Input: part model. Units: mm. Frame: model coordinates. Face numbers are marked on the shaded views. A direction names the side the tool comes from. Give positions to 0.01 mm unless a question says otherwise; leave off trailing zeros. Loops run counter-clockwise (first coordinate to the right, second up) from the corner with the lowest first, then second, coordinate; pieces in that order, holes last. Notation, with made-up numbers: M 55.25,42.25 L 75.25,42.25 A26 cw 75.25,65.25 Z; hole C -6.5,79.25 d5. An arc over 180 degrees is marked long. Use a Markdown table: item, result. Add a question column.
from build123d import *

# Parameters (mm, degrees)
BOSS_EXTRUDE1_DEPTH  = 32.5
SKETCH4_R            = 1.05
BOSS_EXTRUDE2_DEPTH  = 2
SKETCH7_R            = 2.495
WIRE_SPACING2_DEPTH  = 3
SKETCH8_W            = 35
SKETCH8_H            = 37.7
SKETCH8_R            = 2.495
BOSS_EXTRUDE6_DEPTH  = 2
SKETCH5_R            = 1.05
BOSS_EXTRUDE3_DEPTH  = 2
SKETCH9_R            = 2.495
WIRE_SPACING1_DEPTH  = 3
SKETCH10_W           = 35
SKETCH10_H           = 37.7
SKETCH10_R           = 2.495
BOSS_EXTRUDE8_DEPTH  = 2
SKETCH11_R           = 12.5
CUT_EXTRUDE1_DEPTH   = 47.5
CUT_EXTRUDE2_DEPTH   = 47.5
SKETCH13_W           = 45
SKETCH13_H           = 46.5
BOSS_EXTRUDE9_DEPTH  = 17.5
SKETCH15_W           = 12.5
SKETCH15_H           = 46.5
BOSS_EXTRUDE10_DEPTH = 50
SKETCH18_R           = 4
SKETCH18_R_2         = 1.7
BOSS_EXTRUDE11_DEPTH = 46.5
BOSS_EXTRUDE13_DEPTH = 46.5
SKETCH21_W           = 89.912502986
SKETCH21_H           = 37.65
CUT_EXTRUDE3_DEPTH   = 46
CUT_EXTRUDE5_DEPTH   = 47.5
CUT_EXTRUDE4_START   = -50.5000001
CUT_EXTRUDE4_DEPTH   = 101.5000002
CUT_EXTRUDE6_DEPTH   = 53.0000001
BOSS_EXTRUDE14_DEPTH = 46.5
FILLET2_R            = 10
SKETCH29_W           = 2.5
SKETCH29_H           = 42.5
CUT_EXTRUDE8_DEPTH   = 9.427041
FILLET3_R            = 1
SKETCH30_W           = 7.311581117
SKETCH30_H           = 8
CUT_EXTRUDE9_DEPTH   = 22.5


with BuildPart() as part:
    # Sketch2 → Boss-Extrude1 (new body)
    with BuildSketch(Plane(origin=(0, 0, 0), x_dir=(1, 0, 0), z_dir=(0, 1, 0))):
        Polygon((17.5, 0), (17.5, 37.7), (15, 37.7), (15, 2.5), (-15, 2.5), (-15, 37.7), (-17.5, 37.7), (-17.5, 0), align=None)
    extrude(amount=BOSS_EXTRUDE1_DEPTH)

    # Sketch4 → Boss-Extrude2 (add)
    with BuildSketch(Plane.XZ):
        Polygon((-17.5, 0), (-17.5, -7.443777264), (-17.5, -37.7), (-15, -37.7), (-15, -7.5), (15, -7.5), (15, -37.7), (17.5, -37.7), (17.5, -7.443777264), (17.5, 0), align=None)
        with Locations((-10.1889, -4.95)):
            Circle(SKETCH4_R, mode=Mode.SUBTRACT)
        with Locations((10.1889, -4.95)):
            Circle(SKETCH4_R, mode=Mode.SUBTRACT)
    extrude(amount=BOSS_EXTRUDE2_DEPTH)

    # Sketch7 → Wire spacing2 (add)
    with BuildSketch(Plane.XZ.offset(2)):
        Polygon((-17.5, 0), (-17.5, -37.7), (-15, -37.7), (-15, -7.5), (15, -7.5), (15, -37.7), (17.5, -37.7), (17.5, 0), align=None)
        with Locations((-10.1889, -4.95)):
            Circle(SKETCH7_R, mode=Mode.SUBTRACT)
        with Locations((10.1889, -4.95)):
            Circle(SKETCH7_R, mode=Mode.SUBTRACT)
    extrude(amount=WIRE_SPACING2_DEPTH)

    # Sketch8 → Boss-Extrude6 (add)
    with BuildSketch(Plane.XZ.offset(5)):
        with Locations((0, -18.85)):
            Rectangle(SKETCH8_W, SKETCH8_H)
        with Locations((-10.1889, -4.95)):
            Circle(SKETCH8_R, mode=Mode.SUBTRACT)
        with Locations((10.1889, -4.95)):
            Circle(SKETCH8_R, mode=Mode.SUBTRACT)
    extrude(amount=BOSS_EXTRUDE6_DEPTH)

    # Sketch5 → Boss-Extrude3 (add)
    with BuildSketch(Plane(origin=(0, 32.5, 0), x_dir=(1, 0, 0), z_dir=(0, 1, 0))):
        Polygon((-7.439, 10), (-7.439, 2.5), (7.439, 2.5), (7.439, 10), (10.1889, 12), (15, 12), (15, 37.7), (17.5, 37.7), (17.5, 0), (-17.5, 0), (-17.5, 37.7), (-15, 37.7), (-15, 12), (-10.1889, 12), align=None)
        with Locations((-10.1889, 8.7)):
            Circle(SKETCH5_R, mode=Mode.SUBTRACT)
        with Locations((10.1889, 8.7)):
            Circle(SKETCH5_R, mode=Mode.SUBTRACT)
    extrude(amount=BOSS_EXTRUDE3_DEPTH)

    # Sketch9 → Wire spacing1 (add)
    with BuildSketch(Plane(origin=(0, 34.5, 0), x_dir=(1, 0, 0), z_dir=(0, 1, 0))):
        Polygon((-17.5, 0), (-17.5, 37.7), (-15, 37.7), (-15, 12), (-10.1889, 12), (-7.439, 10), (-7.439, 2.5), (7.439, 2.5), (7.439, 10), (10.1889, 12), (15, 12), (15, 37.7), (17.5, 37.7), (17.5, 0), align=None)
        with Locations((-10.1889, 8.7)):
            Circle(SKETCH9_R, mode=Mode.SUBTRACT)
        with Locations((10.1889, 8.7)):
            Circle(SKETCH9_R, mode=Mode.SUBTRACT)
    extrude(amount=WIRE_SPACING1_DEPTH)

    # Sketch10 → Boss-Extrude8 (add)
    with BuildSketch(Plane(origin=(0, 37.5, 0), x_dir=(1, 0, 0), z_dir=(0, 1, 0))):
        with Locations((0, 18.85)):
            Rectangle(SKETCH10_W, SKETCH10_H)
        with Locations((-10.1889, 8.7)):
            Circle(SKETCH10_R, mode=Mode.SUBTRACT)
        with Locations((10.1889, 8.7)):
            Circle(SKETCH10_R, mode=Mode.SUBTRACT)
    extrude(amount=BOSS_EXTRUDE8_DEPTH)

    # Sketch11 → Cut-Extrude1 (cut, through all)
    with BuildSketch(Plane(origin=(0, 39.5, 0), x_dir=(1, 0, 0), z_dir=(0, 1, 0))):
        with Locations((0, 37.7)):
            Circle(SKETCH11_R)
    extrude(amount=-CUT_EXTRUDE1_DEPTH, mode=Mode.SUBTRACT)

    # Sketch12 → Cut-Extrude2 (cut, through all)
    with BuildSketch(Plane.XZ.offset(7)):
        Polygon((0, -25.2), (17.5, -15), (17.5, -47.484525272), align=None)
    extrude(amount=-CUT_EXTRUDE2_DEPTH, mode=Mode.SUBTRACT)

    # Sketch13 → Boss-Extrude9 (add)
    with BuildSketch(Plane.XY):
        with Locations((-5, 16.25)):
            Rectangle(SKETCH13_W, SKETCH13_H)
    extrude(amount=BOSS_EXTRUDE9_DEPTH)

    # Sketch15 → Boss-Extrude10 (add)
    with BuildSketch(Plane(origin=(0, 0, 0), x_dir=(-1, 0, 0), z_dir=(0, 0, -1))):
        with Locations((21.25, 16.25)):
            Rectangle(SKETCH15_W, SKETCH15_H)
    extrude(amount=BOSS_EXTRUDE10_DEPTH)

    # Sketch18 → Boss-Extrude11 (add)
    with BuildSketch(Plane.XZ.offset(7)):
        with BuildLine():
            Line((12.5, 22.5), (12.5, 17.5))
            Line((12.5, 17.5), (-12.5, 17.5))
            Line((-12.5, 17.5), (-12.5, 22.5))
            Line((-12.5, 22.5), (-9.367496998, 30))
            ThreePointArc((-9.367496998, 30), (0, 49.5), (9.367496998, 30))
            Line((9.367496998, 30), (12.5, 22.5))
        make_face()
        with Locations((0, 37.5)):
            Circle(SKETCH18_R, mode=Mode.SUBTRACT)
        with Locations((0, 30.5)):
            Circle(SKETCH18_R_2, mode=Mode.SUBTRACT)
        with Locations((-7, 37.5)):
            Circle(SKETCH18_R_2, mode=Mode.SUBTRACT)
        with Locations((0, 44.5)):
            Circle(SKETCH18_R_2, mode=Mode.SUBTRACT)
        with Locations((7, 37.5)):
            Circle(SKETCH18_R_2, mode=Mode.SUBTRACT)
    extrude(amount=-BOSS_EXTRUDE11_DEPTH)

    # Sketch22 → Boss-Extrude13 (add)
    with BuildSketch(Plane.XZ.offset(7)):
        Polygon((-27.5, 17.5), (-5.066300312, 48.378078928), (-5.066300312, 17.5), align=None)
        Polygon((17.5, 17.5), (6.194336088, 47.777655396), (7.922300343, 17.5), align=None)
    extrude(amount=-BOSS_EXTRUDE13_DEPTH)

    # Sketch21 → Cut-Extrude3 (cut, through all)
    with BuildSketch(Plane.ZY.offset(27.5)):
        with Locations((62.456251493, 16.25)):
            Rectangle(SKETCH21_W, SKETCH21_H)
    extrude(amount=-CUT_EXTRUDE3_DEPTH, mode=Mode.SUBTRACT)

    # Sketch26 → Cut-Extrude5 (cut, through all)
    with BuildSketch(Plane(origin=(0, 39.5, 0), x_dir=(1, 0, 0), z_dir=(0, 1, 0))):
        with BuildLine():
            Line((-27.5, 29.387171818), (-27.5, 50))
            Line((-27.5, 50), (-15, 50))
            add(Edge.make_bspline(
                [(-15, 50), (-23.594741162, 41.153529081), (-27.5, 29.387171818)],
                knots=[0, 0, 0, 1, 1, 1], degree=2))
        make_face()
    extrude(amount=-CUT_EXTRUDE5_DEPTH, mode=Mode.SUBTRACT)

    # Sketch24 → Cut-Extrude4 (cut)
    with BuildSketch(Plane(origin=(0, 0, 0), x_dir=(-1, 0, 0), z_dir=(0, 0, -1)).offset(CUT_EXTRUDE4_START)):
        with BuildLine():
            Line((15, -7), (27.5, -7))
            Line((27.5, -7), (27.5, 16.25))
            add(Edge.make_bspline(
                [(27.5, 16.25), (23.398461901, 3.482399142), (15, -7)],
                knots=[0, 0, 0, 1, 1, 1], degree=2))
        make_face()
    cut_extrude4 = extrude(amount=CUT_EXTRUDE4_DEPTH, mode=Mode.SUBTRACT)

    # Mirror1: Cut-Extrude4 across plane
    add(cut_extrude4.mirror(Plane(origin=(0, 16.25, 0), x_dir=(0, 0, 1), z_dir=(0, -1, 0))), mode=Mode.SUBTRACT)

    # Sketch27 → Cut-Extrude6 (cut, through all)
    with BuildSketch(Plane(origin=(0, 0, -2.5), x_dir=(-1, 0, 0), z_dir=(0, 0, -1))):
        Polygon((-12.5, 26.25), (8.945069205, 16.25), (-12.5, 6.25), align=None)
    extrude(amount=-CUT_EXTRUDE6_DEPTH, mode=Mode.SUBTRACT)

    # Sketch28 → Boss-Extrude14 (add)
    with BuildSketch(Plane(origin=(0, 39.5, 0), x_dir=(1, 0, 0), z_dir=(0, 1, 0))):
        Polygon((-15, 37.7), (-15, 50), (-10, 50), (-10, 47.127040762), (-12.5, 47.127040762), (-12.5, 37.7), align=None)
    extrude(amount=-BOSS_EXTRUDE14_DEPTH)

    # Fillet2
    fillet2_edges = [part.edges().sort_by_distance(p)[0] for p in [
        (-15, 16.25, -50),
    ]]
    fillet(fillet2_edges, radius=FILLET2_R)

    # Sketch29 → Cut-Extrude8 (cut)
    with BuildSketch(Plane.XY.offset(-37.7)):
        with Locations((-13.75, 16.25)):
            Rectangle(SKETCH29_W, SKETCH29_H)
    extrude(amount=-CUT_EXTRUDE8_DEPTH, mode=Mode.SUBTRACT)

    # Fillet3
    fillet3_edges = [part.edges().sort_by_distance(p)[0] for p in [
        (-10, 16.25, -47.127040762),
    ]]
    fillet(fillet3_edges, radius=FILLET3_R)

    # Sketch30 → Cut-Extrude9 (cut)
    with BuildSketch(Plane.XY.offset(-47.127040762)):
        with Locations((-9.844209442, 16.25)):
            Rectangle(SKETCH30_W, SKETCH30_H)
    extrude(amount=-CUT_EXTRUDE9_DEPTH, mode=Mode.SUBTRACT)


solid = part.part
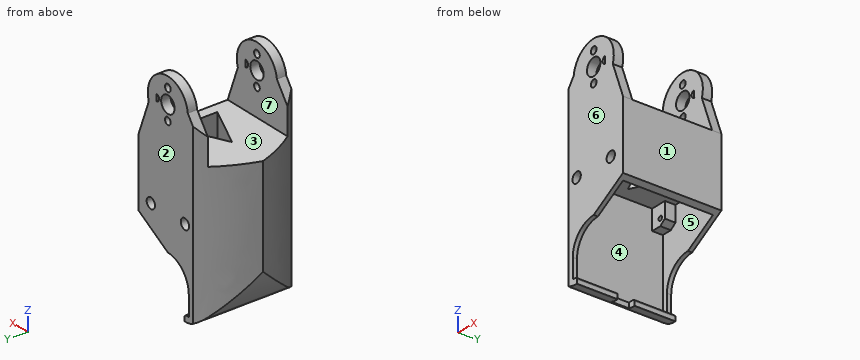
1) Section query B-B, the plane x = -6. Return the cut outline in (y, z) (3 decimals), and give its area (3 significant figures).
2) Contact query for flat-ended pins moving along their axis: P1, Ø8, axis at x = -1.5, y = 5.5, coming from the -Z side; P2, Ø6, axis at y = -1, z = -29.5, coming from the -X side; P3, Ø1.5, axis at x = -8.5, y = 24, coming from the +Z side. Output: stop coordinate, or through.
3) Reachability of the marked faces 5, 6 and 7 from +Z, -Z, +X, -X, +Y, -Y: full face, straight path, thin tool, end or side. Return the list, or none.
4) Pull-direction query (Y, two-part tool) for the marked faces 1, 2, 3 and 4; classes: pulls with the +Y half, pulls with the -Y half, needs draft (parallel to the pull), parting line crosses it, or undercut.
5) Ray query, line 1 (Z direction, x = 0, y = 36); line 2 (Y direction, x = -4, z = -3.5); line 3 (Y direction, x = 1, z = -16). Return the intervals inside material, ascending. Write a range as [from, to].
6) Section query A-A, the plane z = 44.5. Return the cut outline in (x, y) (3 decimals).
Entries:
| question | item | result |
|---|---|---|
| 1 | outline | M -7,-26.734 L -5,-26.734 L -5,-7.5 L 0,-7.5 L 0,-2.5 L 14.877,-2.5 L 14.877,17.5 L -2.575,17.5 L -2.575,47.892 L -7,47.892 Z; M 17.623,-2.5 L 37.5,-2.5 L 37.5,-26.734 L 39.5,-26.734 L 39.5,47.892 L 35.075,47.892 L 35.075,17.5 L 17.623,17.5 Z |
| 1 | area | 1,270 mm² |
| 2 | P1 | stops at z = -2.5 |
| 2 | P2 | stops at x = -21.18 |
| 2 | P3 | stops at z = 17.5 |
| 3 | face 5 | none |
| 3 | face 6 | +Z, -Z, +X, -X, -Y |
| 3 | face 7 | +Z, +X, -X |
| 4 | face 1 | needs draft |
| 4 | face 2 | pulls with the +Y half |
| 4 | face 3 | undercut |
| 4 | face 4 | undercut |
| 5 | line 1 | z = [-2.5, 28.8], [32.2, 33.5], [41.5, 42.8], [46.2, 49.5] |
| 5 | line 2 | y = [-7, 0], [37.5, 39.5] |
| 5 | line 3 | y = [-7, -5], [37.5, 39.5] |
| 6 | outline | M -9.747,-7 L -1.7,-7 L -1.7,-2.575 L -9.747,-2.575 Z; M -9.747,35.075 L -1.7,35.075 L -1.7,39.5 L -9.747,39.5 Z; M 1.7,-7 L 9.747,-7 L 9.747,-2.575 L 1.7,-2.575 Z; M 1.7,35.075 L 9.747,35.075 L 9.747,39.5 L 1.7,39.5 Z |
